Geometry: see drawing. Coordinates: mm, zero at the bounding-box minimum. A direction names the side the tool comes from. Give positions to 0.01 mm unless a question says otherwise; leave off trailing zeros. Order: outer loops, then holes, each group sorted by start corner. A loop starts at its lowest first (then second) coordinate and runs counter-clockwise, first axis right, second up. Notation, with made-up numbers: M 87.25,-37.5 L 125.25,-37.5 A31 cw 125.25,-7.5 Z; hole C 26.25,11 d6. An arc over 180 degrees is marked long. Return JSON: item names as keys, results as strings.
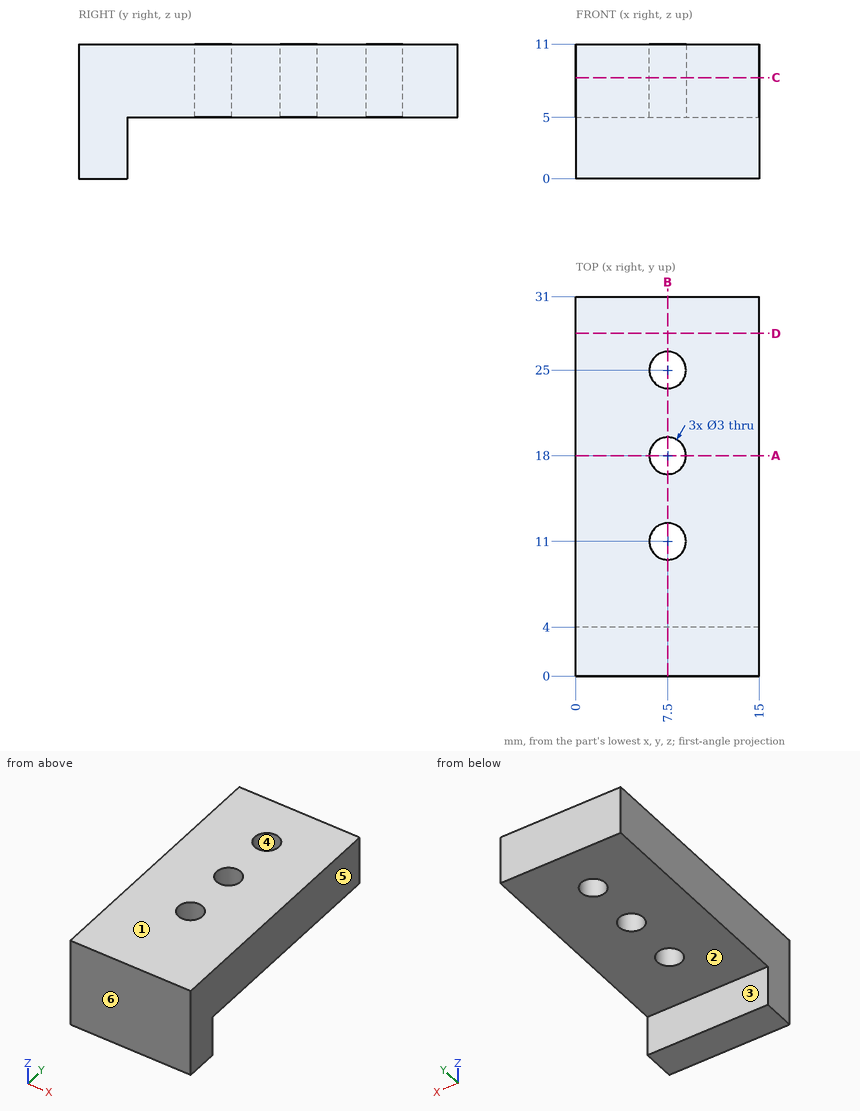
1. Ray query, probe 1 along Y at (x, z) = (7.5, 6.55); probe 2 along Y at (x, z) = (8.5, 7.75); probe 3 along Z at (x, y) = (11.25, 24.5). Return the intervals inside material, ascending.
Evaluation:
{"probe 1": "y = 0 to 9.5, 12.5 to 16.5, 19.5 to 23.5, 26.5 to 31", "probe 2": "y = 0 to 9.88, 12.12 to 16.88, 19.12 to 23.88, 26.12 to 31", "probe 3": "z = 5 to 11"}
2. Set-up query: the marked faces 1 and 2. Return all of +Z, -Z, +X, -X, +Y, -Y with unobstructed straight access to the full face (end or side cutting, diameter ignored); none if empty.
Evaluation:
{"face 1": "+Z, +X, -X, +Y, -Y", "face 2": "-Z, +X, -X, +Y"}
3. Section query A-A (y = 18). Return loops of the section in (x, z).
Evaluation:
{"outline": "M 0,5 L 6,5 L 6,11 L 0,11 Z; M 9,5 L 15,5 L 15,11 L 9,11 Z"}
4. Draft query along Y for the marked faces 3, 4, 5 and 6. Return one class per face: pulls with the +Y half, pulls with the -Y half, needs draft (parallel to the pull), parting line crosses it, or undercut.
Evaluation:
{"face 3": "pulls with the +Y half", "face 4": "undercut", "face 5": "needs draft", "face 6": "pulls with the -Y half"}
5. Section query D-D (y = 28). Return loops of the section in (x, z).
Evaluation:
{"outline": "M 0,5 L 15,5 L 15,11 L 0,11 Z"}
6. First-contact query: pin 1 (1 mm diameter, centred on x = 12, y = 15, fed in from -Z); pin 2 (2.5 mm diameter, centred on x = 8, z = 2, fed in from +Y). Flat tips, straight axial feed; report the tip coordinate or a pass-through.
Evaluation:
{"pin 1": "stops at z = 5", "pin 2": "stops at y = 4"}
7. Section query B-B (x = 7.5). Return loops of the section in (y, z), then the cut area to 3 significant figures.
Evaluation:
{"outline": "M 0,0 L 4,0 L 4,5 L 9.5,5 L 9.5,11 L 0,11 Z; M 12.5,5 L 16.5,5 L 16.5,11 L 12.5,11 Z; M 19.5,5 L 23.5,5 L 23.5,11 L 19.5,11 Z; M 26.5,5 L 31,5 L 31,11 L 26.5,11 Z", "area": "152 mm^2"}
8. Section query C-C (z = 8.25). Return loops of the section in (x, y).
Evaluation:
{"outline": "M 0,0 L 15,0 L 15,31 L 0,31 Z; hole C 7.5,11 d3; hole C 7.5,18 d3; hole C 7.5,25 d3"}
